Can you work these out from the drawing? Everything is in mm from the part's minimum corner. Coordinates: 2 decimals unless noted, no trailing zeros. Order: outer loops, then holes, each group sorted by start corner. A loop starts at its lowest first (then second) coordinate and runs counter-clockwise, first axis right, second up. Notation, with made-up numbers: M -7.5,62.25 L 31.5,62.25 A27 ccw 31.5,99.25 Z; hole C 75,8.5 d9. An arc over 180 degrees is marked long. Answer as a JSON object with one key per item and string values.
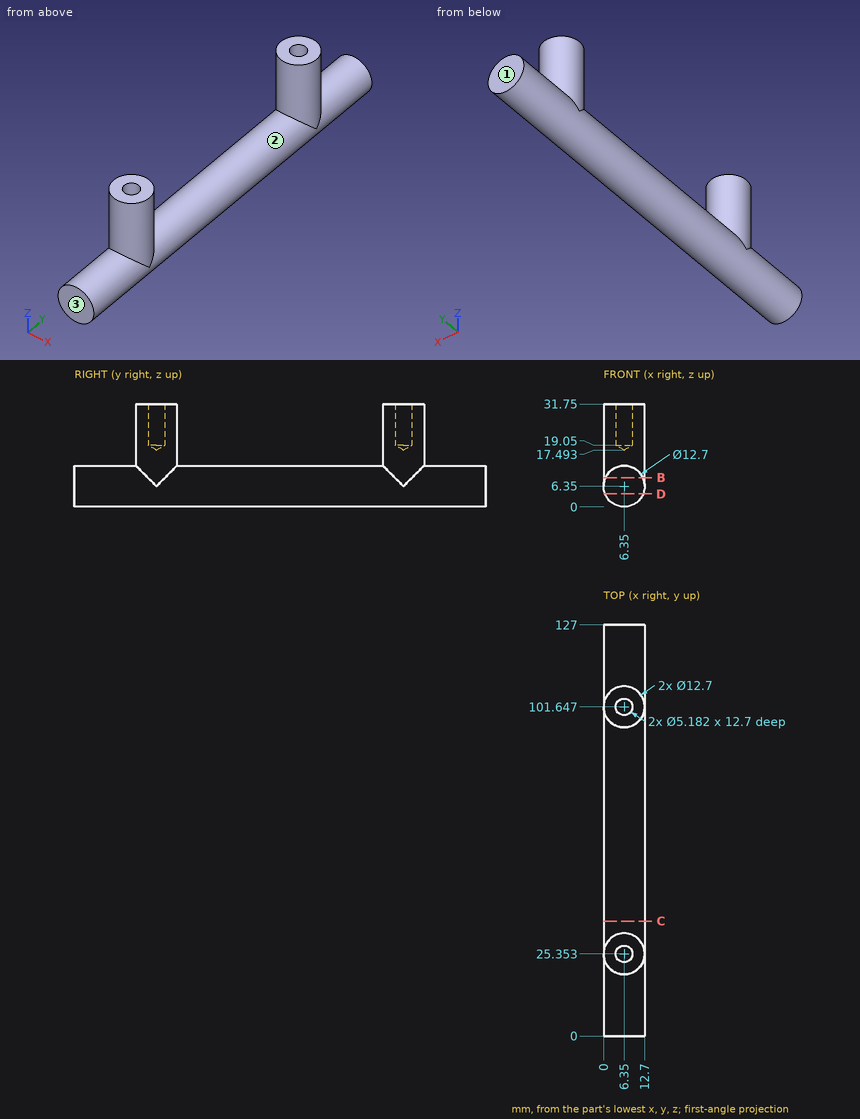
Item 1: I want a section at C-C, the plane y = 35.5. Write out the boundary of the cut face in (x, z), plus the area to 3 significant figures.
Answers follow:
{"outline": "C 6.35,6.35 d12.7", "area": "127 mm^2"}
Item 2: If we mould it in two halves opening along Y, with no side actions, what happens to the marked faces 1, 2 and 3? For each: pulls with the +Y half, pulls with the -Y half, needs draft (parallel to the pull), parting line crosses it, or undercut.
Answers follow:
{"face 1": "pulls with the +Y half", "face 2": "undercut", "face 3": "pulls with the -Y half"}
Item 3: I want a section at B-B, the plane z = 9. Write out the boundary of the cut face in (x, y), plus the area to 3 significant figures.
Answers follow:
{"outline": "M 0.58,0 L 12.12,0 L 12.12,22.7 A6.35 ccw 12.12,28 L 12.12,99 A6.35 ccw 12.12,104.3 L 12.12,127 L 0.58,127 L 0.58,104.3 A6.35 ccw 0.58,99 L 0.58,28 A6.35 ccw 0.58,22.7 Z", "area": "1,470 mm^2"}
Item 4: Please list where these lines run through material, in increasing order: line 1 (Y direction, x = 6.35, z = 28.25); line 2 (Y direction, x = 6.25, z = 15); line 3 (Z direction, x = 6, y = 112).
Answers follow:
{"line 1": "y = 19 to 22.76, 27.94 to 31.7, 95.3 to 99.06, 104.24 to 108", "line 2": "y = 19 to 31.7, 95.3 to 108", "line 3": "z = 0.01 to 12.69"}
Item 5: I want a section at D-D, the plane z = 4. Write out the boundary of the cut face in (x, y).
Answers follow:
{"outline": "M 0.45,0 L 12.25,0 L 12.25,127 L 0.45,127 Z"}
Item 6: I'm going to push flat-ended pins straight in: pin 1 (1.5 mm diameter, centred on x = 5, y = 17.5, fed in from +Z); pin 2 (1 mm diameter, centred on x = 3.5, y = 73, fed in from +Z); pin 3 (2 mm diameter, centred on y = 55.5, z = 12.5, fed in from +X) (1 decimal). Where does each tip first touch, or does it pass through?
Answers follow:
{"pin 1": "stops at z = 12.67", "pin 2": "stops at z = 12.25", "pin 3": "stops at x = 10.1"}
